```python
from build123d import *

# Parameters (mm, degrees)
BOSS_EXTRUDE1_DEPTH     = 15.875
FILLET1_R               = 6.35
CUT_EXTRUDE1_DEPTH      = 1
CUT_EXTRUDE1_DEPTH_BACK = 689.975


with BuildPart() as part:
    # Sketch1 → Boss-Extrude1 (new body)
    with BuildSketch(Plane.XY):
        Polygon((-336.55, -45.4914), (-336.55, -59.7789), (336.55, -59.7789), (336.55, -45.4914), (344.4875, -45.4914), (344.4875, 45.4914), (336.55, 45.4914), (336.55, 59.7789), (-336.55, 59.7789), (-336.55, 45.4914), (-344.4875, 45.4914), (-344.4875, -45.4914), align=None)
    extrude(amount=BOSS_EXTRUDE1_DEPTH)

    # Fillet1
    fillet1_edges = [part.edges().sort_by_distance(p)[0] for p in [
        (-336.55, 45.4914, 7.9375),
        (-336.55, -45.4914, 7.9375),
        (336.55, -45.4914, 7.9375),
        (336.55, 45.4914, 7.9375),
    ]]
    fillet(fillet1_edges, radius=FILLET1_R)

    # Sketch2 → Cut-Extrude1 (cut, two sides)
    with BuildSketch(Plane(origin=(344.4875, 0, 0), x_dir=(0, 0, -1), z_dir=(1, 0, 0))) as cut_extrude1_sk:
        Polygon((0, 59.7789), (-15.875, 56.259497231), (-15.875, 59.7789), align=None)
    extrude(amount=CUT_EXTRUDE1_DEPTH, mode=Mode.SUBTRACT)
    extrude(cut_extrude1_sk.sketch, amount=-CUT_EXTRUDE1_DEPTH_BACK, mode=Mode.SUBTRACT)


solid = part.part
```
The listing builds one solid part. Answer for the finished solid, in the listing's coordinates (mm). Coordinates: 2 decimals unless noted, no trailing zeros. Loops run counter-clockwise (first coordinate to the right, second up) from the corner with the lowest first, then second, coordinate; pieces in that order, holes last. Notation, with made-up numbers: (-17.5, -22) - (39.5, -22) arc R14 cw to (39.5, 1) - close; hole circle Ø2 at (45.25, 53.25). An arc over 180 degrees is marked (long way). Write item = value, one per line.
1) Each of these flat-tipped pins is pushed along its axis until it touches: P1, Ø1, axis at x = -7.5, y = -8, coming from the -Z side; P2, Ø1.7, axis at x = -343.5, z = 7.5, coming from the -Y side; P3, Ø3, axis at x = -208.5, z = 2.5, coming from the +Y side; P4, Ø8.5, axis at y = -57, z = 4.5, coming from the -X side. Where does it stop, or does it pass through?
Responses:
P1 = 0
P2 = -45.5
P3 = 59.56
P4 = -336.55
2) Find the intervals of material crossed by line 1 along Y through (x, z) = (271, 8.25); line 2 along Y through (x, z) = (207, 10); line 3 along X through (y, z) = (50, 2.75), in increasing order.
Responses:
line_1 = -59.78 to 57.95
line_2 = -59.78 to 57.56
line_3 = -336.82 to 336.82
3) Section A-A (z = 12) is taken. Determine the outline of the cut face in (x, y).
Responses:
outline = (-344.49, -45.49) - (-342.9, -45.49) arc R6.35 cw to (-336.55, -51.84) - (-336.55, -59.78) - (336.55, -59.78) - (336.55, -51.84) arc R6.35 cw to (342.9, -45.49) - (344.49, -45.49) - (344.49, 45.49) - (342.9, 45.49) arc R6.35 cw to (336.55, 51.84) - (336.55, 57.12) - (-336.55, 57.12) - (-336.55, 51.84) arc R6.35 cw to (-342.9, 45.49) - (-344.49, 45.49) - close
